Input: part model. Units: mm. Frame: model coordinates. Give positions to 0.01 mm unless a question says otherwise; leave off trailing zeros. Write each loop counter-clockwise with the first axis right and the second up, starting at its lowest first coordinate (ties: lowest second). Pieces come first, ordered by that corner, then holes. Notation, with made-up numbers: M 80.25,88.25 L 104.25,88.25 A14 cw 104.25,101.25 Z; hole C -36,42 d10. An arc over 180 degrees is marked long. Use CSV: the item, a comma, the result in double quotes. Start each with the question number.
from build123d import *

# Parameters (mm, degrees)
SKETCH1_R           = 2.35
BOSS_EXTRUDE1_DEPTH = 7.8


with BuildPart() as part:
    # Sketch1 → Boss-Extrude1 (new body)
    with BuildSketch(Plane(origin=(0, 0, 0), x_dir=(0, 0, -1), z_dir=(1, 0, 0))):
        with BuildLine():
            Line((-40, -3.73), (40, -3.73))
            ThreePointArc((40, -3.73), (43.73, 0), (40, 3.73))
            Line((40, 3.73), (-40, 3.73))
            ThreePointArc((-40, 3.73), (-43.73, 0), (-40, -3.73))
        make_face()
        with Locations((-40, 0)):
            Circle(SKETCH1_R, mode=Mode.SUBTRACT)
        with Locations((-32, 0)):
            Circle(SKETCH1_R, mode=Mode.SUBTRACT)
        with Locations((-24, 0)):
            Circle(SKETCH1_R, mode=Mode.SUBTRACT)
        with Locations((-16, 0)):
            Circle(SKETCH1_R, mode=Mode.SUBTRACT)
        with Locations((-8, 0)):
            Circle(SKETCH1_R, mode=Mode.SUBTRACT)
        Circle(SKETCH1_R, mode=Mode.SUBTRACT)
        with Locations((8, 0)):
            Circle(SKETCH1_R, mode=Mode.SUBTRACT)
        with Locations((16, 0)):
            Circle(SKETCH1_R, mode=Mode.SUBTRACT)
        with Locations((24, 0)):
            Circle(SKETCH1_R, mode=Mode.SUBTRACT)
        with Locations((32, 0)):
            Circle(SKETCH1_R, mode=Mode.SUBTRACT)
        with Locations((40, 0)):
            Circle(SKETCH1_R, mode=Mode.SUBTRACT)
    extrude(amount=BOSS_EXTRUDE1_DEPTH)


solid = part.part
Q1. Section B-B, the plane x = 3.25. Give the number of separate pieces and of enclosed holes in the cut face, and give its area (3 significant figures).
Q2. Pull-direction query (Y, two-part tool) for faces 1 (the cylindrical face through (3.85, -0.08, -43.73)), 2 (the cylindrical face through (3.85, -0.9, 29.83)), 3 (the flat face through (4, 3.73, -1)); classes: released by +Y, released by -Y, zero draft, split by the parting line, or undercut.
Q3. First-contact query: pin 1 Ø1 at (x, y) = (6, 1) entering from -Z. Flat tip, straight axial feed; report the tip coordinate or a pass-through.
Q4. Section A-A, the plane z = 24. Return the cut outline in (x, y), and give its area (3 significant figures).
Q5. Material intervals for L1, parallel to Y at x = 2.75, z = -40; L2, parallel to Y at x = 7, z = 18; L3, parallel to Z at x = 5.5, y = 3.25, sorted ascending. Write a range as [from, to].
Q6. Section D-D, the plane z = 9.5. Return the cut outline in (x, y), and give its area (3 significant figures).
Check result:
1,separate pieces,"1"
1,enclosed holes,"11"
1,area,"450 mm²"
2,face 1,"split by the parting line"
2,face 2,"undercut"
2,face 3,"released by +Y"
3,pin 1,"stops at z = -43.7"
4,outline,"M 0,-3.73 L 7.8,-3.73 L 7.8,-2.35 L 0,-2.35 Z; M 0,2.35 L 7.8,2.35 L 7.8,3.73 L 0,3.73 Z"
4,area,"21.5 mm²"
5,L1,"y = [-3.73, -2.35], [2.35, 3.73]"
5,L2,"y = [-3.73, -1.23], [1.23, 3.73]"
5,L3,"z = [-41.83, 41.83]"
6,outline,"M 0,-3.73 L 7.8,-3.73 L 7.8,-1.81 L 0,-1.81 Z; M 0,1.81 L 7.8,1.81 L 7.8,3.73 L 0,3.73 Z"
6,area,"30.0 mm²"
